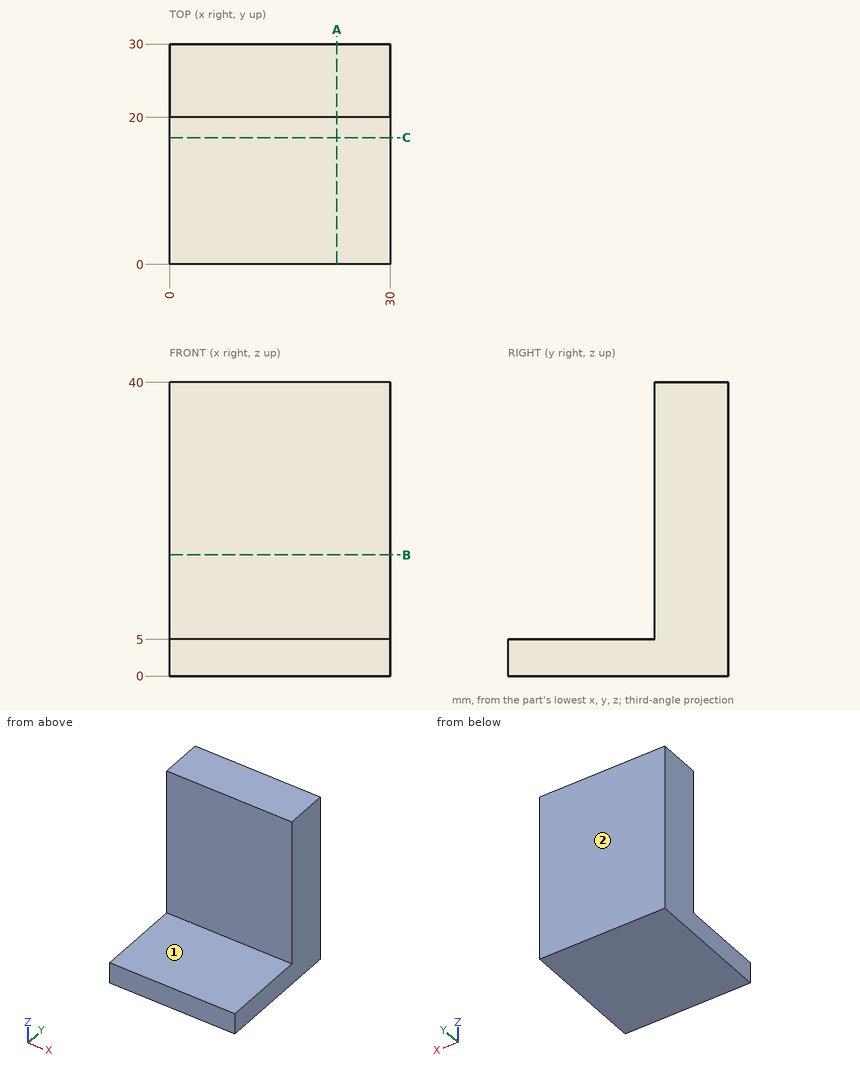
Here's the drawing with two shaded views (mm, measured from the low corner). I have some questions. A direction names the side the tool comes from. Round coordinates to 2 decimals unless told otherwise and drop trailing zeros. Write each loop counter-clockwise with the first axis right and the second up, starting at its lowest first coordinate (ties: lowest second). Pieces come first, ordered by that corner, then holes. Notation, with made-up numbers: M 76,83.5 L 135,83.5 A27 ccw 135,120.5 Z; hole C -30.75,-31 d5. An arc over 180 degrees is marked long. Write each question's results on one line, items separated by ' | '. Start each with the question number.
1. On a 3-axis mill with a long thin cutter (end or side, diameter ignored), from which of +Z, -Z, +X, -X, +Y, -Y can I reach the whole of each face in a straight line? I mean the marked faces 1 and 2. Say none if no direction works.
2. I need wall thicknesses on L1, parallel to Y at x = 19.5, z = 20; L2, parallel to Z at x = 19, y = 2.75. Which ranges of each line are inside material? Lowest first, please. Write a range as from..to.
3. I'm going to push a flat-ended pin straight in: pin 1 Ø10 at (x, z) = (10, 11) entering from -Y. Where does the tip first touch, or does it pass through?
4. Imagine slicing it at A-A on x = 22.75. List the corners of the cut face in (y, z) for me, and give its area (3 significant figures).
5. Imagine slicing it at B-B on z = 16.5. List the corners of the cut face in (x, y) for me.
6. Imagine slicing it at C-C on y = 17.25. List the corners of the cut face in (x, z) for me, and give its area (3 significant figures).
Result sheet:
1) face 1: +Z, +X, -X, -Y | face 2: +Z, -Z, +X, -X, +Y
2) L1: y = 20..30 | L2: z = 0..5
3) pin 1: stops at y = 20
4) outline: M 0,0 L 30,0 L 30,40 L 20,40 L 20,5 L 0,5 Z | area: 500 mm^2
5) outline: M 0,20 L 30,20 L 30,30 L 0,30 Z
6) outline: M 0,0 L 30,0 L 30,5 L 0,5 Z | area: 150 mm^2
